Could you check a few things on this drawing? It's one solid part, dimensions in mm from its lowest x, y, z. A direction names the side the tool comes from. Round coordinates to 2 decimals unless told otherwise and drop trailing zeros. Write each loop counter-clockwise with the first axis right and the second up, starting at its lowest first coordinate (ties: lowest second). Pieces come first, ordered by that corner, then holes. Notation, with made-up numbers: (21, 57) -> (33, 57) arc R6 ccw to (33, 61) -> close; hole circle Ø6 at (21.25, 6.25). An arc over 180 degrees is marked (long way). Return JSON: item names as keys, results as strings.
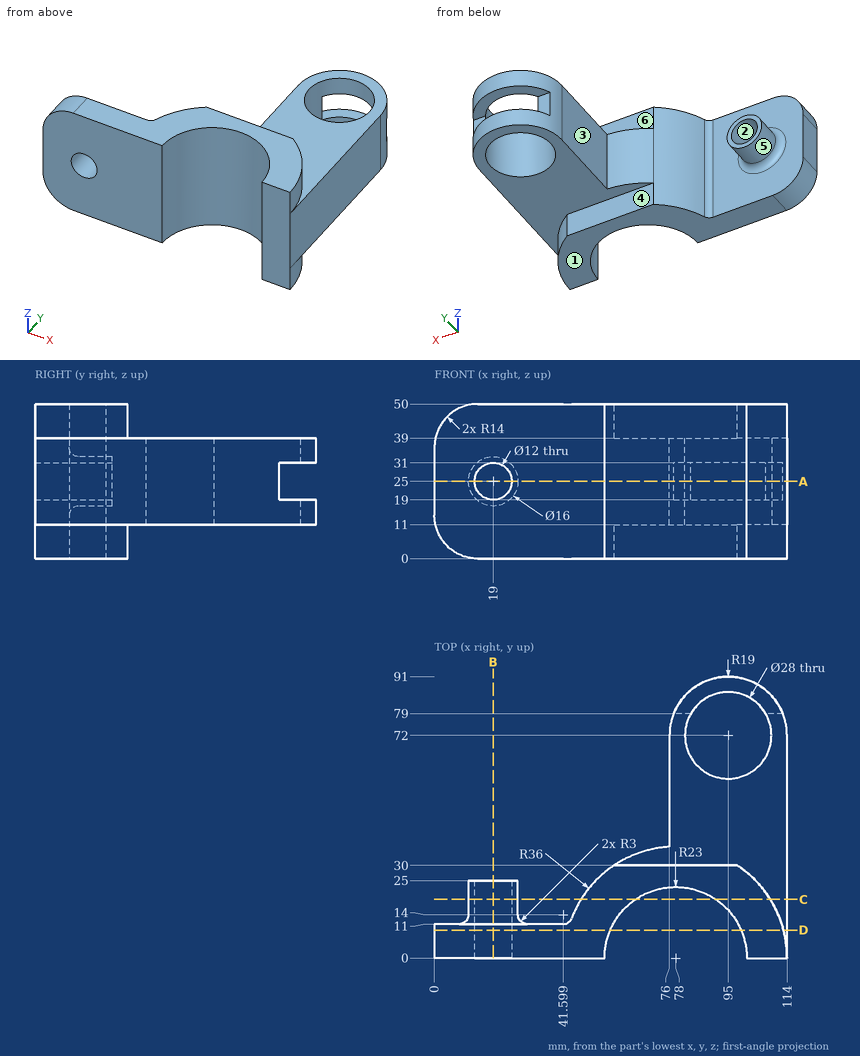
1) If I drill on probe 1 along X at (y, z) = (71.5, 14.5); probe 2 along Z at (x, y) = (19, 7.75); probe 3 along Z at (x, y) = (19, 18), over which ranges is the centre line in solid material (lowest first)? Write a range as [from, to].
Return value:
{"probe 1": "[76, 81.01], [108.99, 114]", "probe 2": "[0, 19], [31, 50]", "probe 3": "[17, 19], [31, 33]"}
2) For the marked faces 4, 5 and 6, which set-ups out of +Z, -Z, +X, -X, +Y, -Y let a thin tool reach every point of the face, with its end or its side?
Return value:
{"face 4": "-Z, +X, -X, +Y", "face 5": "+Y", "face 6": "+Z, +X, -X, +Y"}
3) Will these pins go through, and if not, where does the flat tip stop? pin 1 Ø21 at (x, z) = (30, 27) entering from +Y; pin 2 Ø12 at (x, z) = (87.5, 6) entering from +Y; pin 3 Ø6 at (x, y) = (101.5, 84.5) entering from -Z; pin 4 Ø11 at (x, z) = (19, 25) entering from -Y.
Return value:
{"pin 1": "y = 25", "pin 2": "y = 90.53", "pin 3": "z = 11", "pin 4": "through"}
4) I want a section at D-D, the plane y = 9. Please give me the cut outline in (x, z).
Return value:
{"outline": "(0, 14) arc R14 ccw to (14, 0) -> (56.83, 0) -> (56.83, 50) -> (14, 50) arc R14 ccw to (0, 36) -> close; (99.17, 0) -> (112.86, 0) -> (112.86, 11) -> (114, 11) -> (114, 39) -> (112.86, 39) -> (112.86, 50) -> (99.17, 50) -> close; hole circle Ø12 at (19, 25)"}
5) I want a section at B-B, the plane x = 19. Please give me the cut outline in (y, z).
Return value:
{"outline": "(0, 0) -> (11, 0) -> (11, 14) arc R3 cw to (14, 17) -> (25, 17) -> (25, 19) -> (0, 19) -> close; (0, 31) -> (25, 31) -> (25, 33) -> (14, 33) arc R3 cw to (11, 36) -> (11, 50) -> (0, 50) -> close"}
6) Thinking about a two-plate mould opening in X: for the marked faces 1, 2 and 3, which applies, pulls with the +X half, pulls with the -X half, needs draft (parallel to the pull), parting line crosses it, or undercut?
Return value:
{"face 1": "needs draft", "face 2": "undercut", "face 3": "pulls with the -X half"}
7) I want a section at A-A, the plane z = 25. Please give me the cut outline in (x, y) (1 decimal), and give its area (3 significant figures).
Return value:
{"outline": "(0, 0) -> (13, 0) -> (13, 25) -> (11, 25) -> (11, 14) arc R3 cw to (8, 11) -> (0, 11) -> close; (25, 0) -> (55, 0) arc R23 cw to (101, 0) -> (114, 0) -> (114, 72) arc R19 ccw to (112.7, 79) -> (107.1, 79) arc R14 cw (long way) to (82.9, 79) -> (77.3, 79) arc R19 ccw to (76, 72) -> (76, 35.9) arc R36 ccw to (44.4, 12.9) arc R3 cw to (41.6, 11) -> (30, 11) arc R3 cw to (27, 14) -> (27, 25) -> (25, 25) -> close", "area": "3,010 mm²"}
8) I want a section at C-C, the plane y = 19. Please give me the cut outline in (x, z), and give its area (3 significant figures).
Return value:
{"outline": "circle Ø16 at (19, 25); (47.42, 0) -> (65.04, 0) -> (65.04, 50) -> (47.42, 50) -> close; (90.96, 0) -> (108.58, 0) -> (108.58, 11) -> (114, 11) -> (114, 39) -> (108.58, 39) -> (108.58, 50) -> (90.96, 50) -> close; hole circle Ø12 at (19, 25)", "area": "2,000 mm²"}
